For this review, take the finished solid that the model builds, in its own axes (mm). A direction names the side the tool comes from. Coordinates: 2 decimals unless noted, no trailing zeros. Write each loop counter-clockwise with the first axis right and the second up, starting at its lowest first coordinate (ties: lowest second). Pieces come first, ordered by that corner, then holes.
```python
from build123d import *

# Parameters (mm, degrees)
BOSS_EXTRUDE1_DEPTH = 56
SKETCH3_W           = 16
SKETCH3_H           = 28
CUT_EXTRUDE1_DEPTH  = 61.057795506


with BuildPart() as part:
    # Sketch2 → Boss-Extrude1 (new body)
    with BuildSketch(Plane.XY):
        with BuildLine():
            ThreePointArc((-52.370168415, 4.5), (-50.955954852, 5.085786438), (-50.370168415, 6.5))
            Line((-50.370168415, 6.5), (-50.370168415, 9.5))
            ThreePointArc((-50.370168415, 9.5), (-50.955954852, 10.914213562), (-52.370168415, 11.5))
            Line((-52.370168415, 11.5), (-57.370168415, 11.5))
            Line((-57.370168415, 11.5), (-57.370168415, 13.5))
            Line((-57.370168415, 13.5), (-52.370168415, 13.5))
            ThreePointArc((-52.370168415, 13.5), (-49.54174129, 12.328427125), (-48.370168415, 9.5))
            Line((-48.370168415, 9.5), (-48.370168415, 6.204424851))
            ThreePointArc((-48.370168415, 6.204424851), (-49.54174129, 3.375997726), (-52.370168415, 2.204424851))
            Line((-52.370168415, 2.204424851), (-57.370168415, 2.204424851))
            Line((-57.370168415, 2.204424851), (-57.370168415, -2.795575149))
            Line((-57.370168415, -2.795575149), (-52.370168415, -2.795575149))
            ThreePointArc((-52.370168415, -2.795575149), (-49.54174129, -3.967148025), (-48.370168415, -6.795575149))
            Line((-48.370168415, -6.795575149), (-48.370168415, -12.091150299))
            Line((-48.370168415, -12.091150299), (-43.370168415, -12.93073765))
            Line((-43.370168415, -12.93073765), (-43.370168415, -14.660791284))
            Line((-43.370168415, -14.660791284), (-50.370168415, -13.5))
            Line((-50.370168415, -13.5), (-50.370168415, -6.5))
            ThreePointArc((-50.370168415, -6.5), (-50.955954852, -5.085786438), (-52.370168415, -4.5))
            Line((-52.370168415, -4.5), (-57.370168415, -4.5))
            ThreePointArc((-57.370168415, -4.5), (-58.784381977, -3.914213562), (-59.370168415, -2.5))
            Line((-59.370168415, -2.5), (-59.370168415, 2.5))
            ThreePointArc((-59.370168415, 2.5), (-58.784381977, 3.914213562), (-57.370168415, 4.5))
            Line((-57.370168415, 4.5), (-52.370168415, 4.5))
        make_face()
    extrude(amount=BOSS_EXTRUDE1_DEPTH)

    # Sketch3 → Cut-Extrude1 (cut, through all)
    with BuildSketch(Plane.ZY.offset(59.370168415)):
        with Locations((28, -2.5)):
            Rectangle(SKETCH3_W, SKETCH3_H)
    extrude(amount=-CUT_EXTRUDE1_DEPTH, mode=Mode.SUBTRACT)


solid = part.part
```
Q1. Draft analysis for pull direction Z (two halves, no side actions). For faces 6 (the flat face through (-51, -4, 20)), 7 (the flat face through (-51, 3, 56)), 8 (the cylindrical face through (-50.94, 10.9, 9.86)), state which applies: +Z half, -Z half, draft (parallel to the pull), parting line (faces both ways), or undercut.
Ans:
face 6: undercut
face 7: +Z half
face 8: draft
Q2. Add section B-B (x = -54.75). State the section outline as (y, z) points, then the cut area to 3 significant figures.
Ans:
outline: (-4.5, 0) - (-2.8, 0) - (-2.8, 20) - (-4.5, 20) - close; (-4.5, 36) - (-2.8, 36) - (-2.8, 56) - (-4.5, 56) - close; (2.2, 0) - (4.5, 0) - (4.5, 20) - (2.2, 20) - close; (2.2, 36) - (4.5, 36) - (4.5, 56) - (2.2, 56) - close; (11.5, 0) - (13.5, 0) - (13.5, 56) - (11.5, 56) - close
area: 272 mm2
Q3. Clearance check with flat-ended pins moving along their axes: pin 1 Ø4 at (x, z) = (-51, 37) entering from -Y; pin 2 Ø5.5 at (y, z) = (-1.5, 41) entering from +X; pin 3 Ø3.5 at (y, z) = (7.5, 10) entering from +X; pin 4 Ø1.5 at (x, z) = (-52, 40) entering from +Y. State where each tip first meets the part, or that it passes through.
Ans:
pin 1: stops at y = -13.73
pin 2: stops at x = -49.28
pin 3: stops at x = -48.37
pin 4: stops at y = 13.5
Q4. Tool access review of faces 1 (the flat face through (-55, 2.204, 46)), 2 (the flat face through (-51, -4, 36)), 3 (the flat face through (-48.37, 8, 46)), 4 (the flat face through (-50.37, -10, 46)), 5 (the flat face through (-55, 4.5, 10)): name each direction out of +Z, -Z, +X, -X, +Y, -Y from which nothing blocks a thin tool from reaching the whole face with its end or side.
Ans:
face 1: +Z, -Z, +X
face 2: +X, -X, -Y
face 3: +Z, -Z, +X, +Y
face 4: +Z, -Z, -X, -Y
face 5: +Z, -Z, -X
Q5. For probe 1 along Y at (x, z) = (-54, 45); probe 2 along Z at (x, y) = (-51.75, -4.5); probe 3 along Y at (x, z) = (-51, 9), list the stretches that pass through material, from the lowest coordinate up.
Ans:
probe 1: y = -4.5 to -2.8, 2.2 to 4.5, 11.5 to 13.5
probe 2: z = 0 to 20, 36 to 56
probe 3: y = -5.04 to -3.04, 2.45 to 5.04, 10.96 to 13.26
Q6. Add section A-A (y = 0.25). State the section outline as (x, z) points.
Ans:
outline: (-59.37, 0) - (-57.37, 0) - (-57.37, 20) - (-59.37, 20) - close; (-59.37, 36) - (-57.37, 36) - (-57.37, 56) - (-59.37, 56) - close
Q7. Add section C-C (z = 7.5). State the section outline as (x, y) points, then the cut area to 3 significant figures.
Ans:
outline: (-59.37, -2.5) arc R2 ccw to (-57.37, -4.5) - (-52.37, -4.5) arc R2 cw to (-50.37, -6.5) - (-50.37, -13.5) - (-43.37, -14.66) - (-43.37, -12.93) - (-48.37, -12.09) - (-48.37, -6.8) arc R4 ccw to (-52.37, -2.8) - (-57.37, -2.8) - (-57.37, 2.2) - (-52.37, 2.2) arc R4 ccw to (-48.37, 6.2) - (-48.37, 9.5) arc R4 ccw to (-52.37, 13.5) - (-57.37, 13.5) - (-57.37, 11.5) - (-52.37, 11.5) arc R2 cw to (-50.37, 9.5) - (-50.37, 6.5) arc R2 cw to (-52.37, 4.5) - (-57.37, 4.5) arc R2 ccw to (-59.37, 2.5) - close
area: 104 mm2
Q8. Add section D-D (x = -45). State the section outline as (y, z) points, then the cut area to 3 significant figures.
Ans:
outline: (-14.39, 0) - (-12.66, 0) - (-12.66, 20) - (-14.39, 20) - close; (-14.39, 36) - (-12.66, 36) - (-12.66, 56) - (-14.39, 56) - close
area: 69.3 mm2
